Model file for the job. Use its own axes, mm. Round coordinates to 2 decimals unless told otherwise and drop trailing zeros. Order: outer loops, then holes, each group sorted by start corner. A loop starts at its lowest first (then second) coordinate and runs counter-clockwise, first axis right, second up. Notation, with made-up numbers: (42, -12.5) -> (49, -12.5) arc R14 cw to (49, 2.5) -> close; hole circle Ø3 at (69.25, 24). An arc over 180 degrees is marked (long way). Answer as CSV lines item,"result".
```python
from build123d import *

# Parameters (mm, degrees)
F0_R     = 17.081459
F1_DEPTH = 12.7
F2_SIZE  = 5.08
F3_SIZE  = 5.08


with BuildPart() as f1:
    # F0 (on Front) → F1 (new body)
    with BuildSketch(Plane.XZ):
        Polygon((-17.124444, 15.109803), (-52.100205, 0), (-17.124444, -15.109803), (0, -49.144541), (17.124444, -15.109803), (52.100205, 0), (17.124444, 15.109803), (0, 49.144541), align=None)
        Circle(F0_R, mode=Mode.SUBTRACT)
    extrude(amount=F1_DEPTH)

    # F2
    f2_edges = [f1.edges().sort_by_distance(p)[0] for p in [
        (-34.612325, -12.7, -7.554901),
        (-34.612325, -12.7, 7.554901),
        (-8.562222, -12.7, 32.127172),
        (8.562222, -12.7, 32.127172),
        (34.612325, -12.7, 7.554901),
        (34.612325, -12.7, -7.554901),
        (8.562222, -12.7, -32.127172),
        (-8.562222, -12.7, -32.127172),
    ]]
    chamfer(f2_edges, length=F2_SIZE)

    # F3
    f3_edges = [f1.edges().sort_by_distance(p)[0] for p in [
        (8.562222, 0, 32.127172),
        (-8.562222, 0, 32.127172),
        (-34.612325, 0, 7.554901),
        (-34.612325, 0, -7.554901),
        (-8.562222, 0, -32.127172),
        (8.562222, 0, -32.127172),
        (34.612325, 0, -7.554901),
        (34.612325, 0, 7.554901),
    ]]
    chamfer(f3_edges, length=F3_SIZE)


solid = f1.part
```
Q1. Saw through at D-D (x = 27). Write the cut outline in (y, z), plus the area to 3 significant figures.
Checks:
outline,"(-12.7, -5.31) -> (-7.62, -10.84) -> (-5.08, -10.84) -> (0, -5.31) -> (0, 5.31) -> (-5.08, 10.84) -> (-7.62, 10.84) -> (-12.7, 5.31) -> close"
area,"219 mm²"
Q2. Flat gauge pins, fed straight in: pin 1 (5 mm diameter, centred on x = -30, y = -11, fed in from -Z); pin 2 (3 mm diameter, centred on y = -1.5, z = -19, fed in from -X); pin 3 (1 mm diameter, centred on x = -40.5, y = -6, fed in from -Z). Where does each tip first touch, or does it go through?
Checks:
pin 1,"z = -8.8"
pin 2,"x = -13"
pin 3,"z = -5.23"
Q3. Wall check: L1, parallel to X at y = -7, z = 9; L2, parallel to Z at x = 9.5, y = -3.25; L3, parallel to X at y = -10.5, z = 27.5. Give the ranges that are in metal, low to high. Write a range as [from, to].
Checks:
L1,"[-31.27, -14.52], [14.52, 31.27]"
L2,"[-26.19, -14.2], [14.2, 26.19]"
L3,"[-7.67, 7.67]"
Q4. Saw through at A-A (z = 13.5). Write the cut outline in (x, y).
Checks:
outline,"(-20.85, -7.62) -> (-15.61, -9.7) -> (-12.25, -12.7) -> (-10.47, -12.7) -> (-10.47, 0) -> (-12.25, 0) -> (-15.61, -3) -> (-20.85, -5.08) -> close; (10.47, -12.7) -> (12.25, -12.7) -> (15.61, -9.7) -> (20.85, -7.62) -> (20.85, -5.08) -> (15.61, -3) -> (12.25, 0) -> (10.47, 0) -> close"
Q5. Saw through at B-B (x = 15). Write the cut outline in (y, z).
Checks:
outline,"(-12.7, -10.49) -> (-10.53, -12.86) -> (-7.62, -19.33) -> (-5.08, -19.33) -> (-2.17, -12.86) -> (0, -10.49) -> (0, -8.17) -> (-12.7, -8.17) -> close; (-12.7, 8.17) -> (0, 8.17) -> (0, 10.49) -> (-2.17, 12.86) -> (-5.08, 19.33) -> (-7.62, 19.33) -> (-10.53, 12.86) -> (-12.7, 10.49) -> close"
Q6. Saw through at C-C (y = -11.25). Write the cut outline in (x, z).
Checks:
outline,"(-42.95, 0) -> (-14.47, -12.3) -> (0, -41.07) -> (14.47, -12.3) -> (42.95, 0) -> (14.47, 12.3) -> (0, 41.07) -> (-14.47, 12.3) -> close; hole circle Ø34.16 at (0, 0)"
